```python
from build123d import *

# Parameters (mm, degrees)
BOSS_EXTRUDE1_DEPTH = 3
SKETCH2_W           = 38
SKETCH2_H           = 10
BOSS_EXTRUDE2_DEPTH = 3


with BuildPart() as part:
    # Sketch1 → Boss-Extrude1 (new body)
    with BuildSketch(Plane.XY):
        with BuildLine():
            ThreePointArc((-19, 76.795454546), (-12.552472511, 88.534441856), (0, 93.204545458))
            Line((0, 93.204545458), (0, 102))
            ThreePointArc((0, 102.000000004), (-19.799000732, 93.798979019), (-28, 73.999969292))
            Line((-28, 73.999969292), (-28, 68))
            Line((-28, 68), (-19, 68))
            Line((-19, 68), (-19, 76.795454546))
        make_face()
        with BuildLine():
            Line((0, 102), (0, 93.204545458))
            ThreePointArc((0, 93.204545458), (12.552472511, 88.534441856), (19, 76.795454546))
            Line((19, 76.795454546), (19, 68))
            Line((19, 68), (28, 68))
            Line((28, 68), (28, 73.999969292))
            ThreePointArc((28, 73.999969292), (19.799000732, 93.798979019), (0, 102.000000004))
        make_face()
        Polygon((-19, -1), (-19, 5), (-19, 68), (-28, 68), (-28, 62), (-25, 62), (-25, 5), (-28, 5), (-28, -1), align=None)
        Polygon((19, 68), (19, 5), (19, -1), (28, -1), (28, 5), (25, 5), (25, 62), (28, 62), (28, 68), align=None)
    extrude(amount=BOSS_EXTRUDE1_DEPTH)

    # Sketch2 → Boss-Extrude2 (add)
    with BuildSketch(Plane.XY.offset(3)):
        with Locations((0, 4)):
            Rectangle(SKETCH2_W, SKETCH2_H)
    extrude(amount=-BOSS_EXTRUDE2_DEPTH)


solid = part.part
```
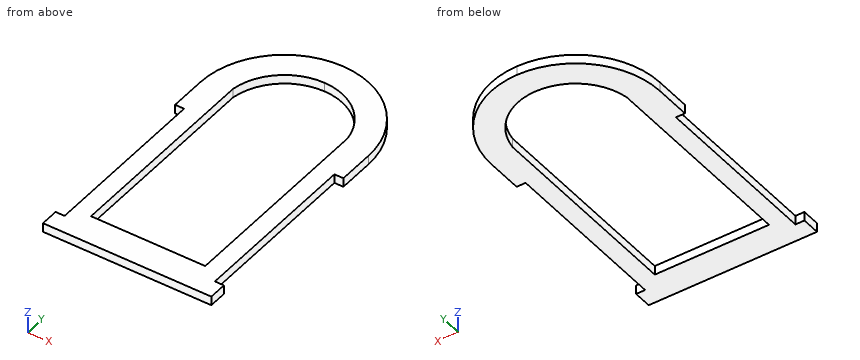
The listing builds one solid part. Answer for the finished solid, in the listing's coordinates (mm). Round coordinates to 2 decimals unless told otherwise and drop trailing zeros. Write each loop counter-clockwise with the first axis right and the second up, starting at its lowest first coordinate (ties: lowest second). Pieces come first, ordered by that corner, then holes. Notation, with made-up numbers: (79.25, -12.75) -> (84.25, -12.75) arc R10 cw to (84.25, 0.25) -> close; hole circle Ø6 at (-29, -28.5). An arc over 180 degrees is marked (long way). Use CSV: the item, a comma, the result in double quotes. Start each with the question number.
(1) Section A-A on z = 1.7 is taken. Give the vertices of the cut face in (x, y).
(2) Section B-B on y = 54.5 is taken. Give the vertices of the cut face in (x, z), then the cut area to 3 significant figures.
(3) Each of these flat-tipped pins is pushed along its axis until it touches: pin 1 (1.5 mm diameter, centred on y = 25, z = 2, fed in from -X); pin 2 (0.9 mm diameter, centred on y = 34.5, z = 1, fed in from +X); pin 3 (1.5 mm diameter, centred on y = 91, z = 2, fed in from -X). Where does it stop, or does it pass through?
(4) Section C-C on x = 1 is taken. Give the vertices of the cut face in (y, z).
(5) Consider L1, parallel to X at y = 68, z = 1.9; L2, parallel to X at y = 24.5, z = 0.55; L3, parallel to Y at x = 14, z = 1.65. Determine where each line is inside the solid, lowest interval first. Write a range as from..to.
A:
1,outline,"(-28, -1) -> (28, -1) -> (28, 5) -> (25, 5) -> (25, 62) -> (28, 62) -> (28, 74) arc R28 ccw to (-28, 74) -> (-28, 62) -> (-25, 62) -> (-25, 5) -> (-28, 5) -> close; hole (-19, 9) -> (19, 9) -> (19, 76.8) arc R19.2 ccw to (-19, 76.8) -> close"
2,outline,"(-25, 0) -> (-19, 0) -> (-19, 3) -> (-25, 3) -> close; (19, 0) -> (25, 0) -> (25, 3) -> (19, 3) -> close"
2,area,"36.0 mm²"
3,pin 1,"stops at x = -25"
3,pin 2,"stops at x = 25"
3,pin 3,"stops at x = -22.8"
4,outline,"(-1, 0) -> (9, 0) -> (9, 3) -> (-1, 3) -> close; (93.18, 0) -> (101.98, 0) -> (101.98, 3) -> (93.18, 3) -> close"
5,L1,"x = -28..-19, 19..28"
5,L2,"x = -25..-19, 19..25"
5,L3,"y = -1..9, 87.15..98.25"
